Here's how the part is built. I have some questions about the finished solid (model axes, mm). A direction names the side the tool comes from. Coordinates: 2 decimals unless noted, no trailing zeros. Write each loop counter-clockwise with the first axis right and the second up, starting at its lowest first coordinate (ties: lowest second). Pieces come first, ordered by that corner, then holes.
Item 1: I'm going to push flat-ended pins straight in: P1, Ø5, axis at x = -108, z = -46.5, coming from the +Y side; P2, Ø12, axis at y = -65.5, z = -42, coming from the +X side; P3, Ø1.8, axis at x = -113, y = -22.5, coming from the +Z side; P4, Ø5, axis at x = -15.5, z = -22.5, coming from the +Y side. Where does each tip first touch, or does it pass through?
Item 2: I want a section at C-C (y = -14). Please give me the cut outline in (x, z), and give its area (3 significant figures).
Item 3: I want a section at A-A (z = -36). Count the separate pieces of the cut face and the enclosed holes in it, and give its area (3 significant figures).
Item 4: For faces 4 (the face through (-70, -11, -65)), 5 (the face through (-134, -3, -35)), 6 (the face through (-131, -12, -43)), 7 (the face through (-99, -1.8, -62)), 8 (the face through (-73.6, -61.9, -29.09)), which set-ups out of +Z, -Z, +X, -X, +Y, -Y let a thin tool reach every point of the face, with its end or its side?
Item 5: I want a section at B-B (x = -50). Please give me the cut outline in (y, z).
Item 6: I want a section at D-D (y = -44). Please give me the cut outline in (x, z), and give its area (3 significant figures).
Item 7: Please list where these lines run through material, in increasing order: line 1 (Y direction, x = -127, z = -37.5); line 2 (X direction, y = -7, z = -15); line 3 (Z direction, x = -83, y = -13).
Item 8: If we mould it in two halves opening along Y, with no side actions, what happens to faces 1 (the face through (-73, -18.5, -33)), 2 (the face through (0, -10, -35)), 3 (the face through (-68, 0, -37))? For each: pulls with the +Y half, pulls with the -Y half, needs draft (parallel to the pull), parting line crosses it, or undercut.
from build123d import *

# Parameters (mm, degrees)
MAIN_BODY_DEPTH     = 16
SKETCH8_W           = 134
SKETCH8_H           = 4
COVER_DEPTH         = 72
SKETCH20_W          = 116
SKETCH20_H          = 14
CRYSTAL_SLOT_DEPTH  = 65
SKETCH9_W           = 14
SKETCH9_H           = 14
SIPM_WINDOW_DEPTH   = 7
SKETCH10_R          = 23
SKETCH10_R_2        = 20
TUBE_ADAPTER_DEPTH  = 85
SKETCH21_W          = 54
SKETCH21_H          = 54
FILTER_SLOT_DEPTH   = 2.7
SKETCH24_W          = 49
SKETCH24_H          = 49
FILTER_WINDOW_DEPTH = 1.8
WIRE_SLOT_REACH     = 146
SKETCH25_W          = 25
SKETCH25_H          = 9


with BuildPart() as part:
    # Sketch5 → Main Body (new body)
    with BuildSketch(Plane(origin=(0, 0, 0), x_dir=(1, 0, 0), z_dir=(0, 1, 0))):
        Polygon((-134, 0), (-124, 0), (-1.95326153, 0), (0, 0), (0, 72), (-134, 72), align=None)
    extrude(amount=-MAIN_BODY_DEPTH)

    # Sketch8 → Cover (add)
    with BuildSketch(Plane.XY):
        with Locations((-67, -18)):
            Rectangle(SKETCH8_W, SKETCH8_H)
    extrude(amount=-COVER_DEPTH)

    # Sketch20 → Crystal Slot (cut)
    with BuildSketch(Plane.XY):
        with Locations((-69, -11.5)):
            Rectangle(SKETCH20_W, SKETCH20_H)
    extrude(amount=-CRYSTAL_SLOT_DEPTH, mode=Mode.SUBTRACT)

    # Sketch9 → SiPM Window (cut)
    with BuildSketch(Plane.ZY.offset(134)):
        with Locations((-36, -11.5)):
            Rectangle(SKETCH9_W, SKETCH9_H)
    extrude(amount=-SIPM_WINDOW_DEPTH, mode=Mode.SUBTRACT)

    # Sketch10 → Tube Adapter (add)
    with BuildSketch(Plane.XZ.offset(20)):
        with Locations((-95.536800003, -36)):
            Circle(SKETCH10_R)
        with Locations((-95.536800003, -36)):
            Circle(SKETCH10_R_2, mode=Mode.SUBTRACT)
    extrude(amount=TUBE_ADAPTER_DEPTH)

    # Sketch21 → Filter Slot (cut)
    with BuildSketch(Plane.XZ.offset(4.5)):
        with Locations((-40.5, -36)):
            Rectangle(SKETCH21_W, SKETCH21_H)
        with Locations((-97, -36)):
            Rectangle(SKETCH21_W, SKETCH21_H)
    extrude(amount=-FILTER_SLOT_DEPTH, mode=Mode.SUBTRACT)

    # Sketch24 → Filter Window (cut)
    with BuildSketch(Plane.XZ.offset(1.8)):
        with Locations((-40.5, -36)):
            Rectangle(SKETCH24_W, SKETCH24_H)
        with Locations((-97, -36)):
            Rectangle(SKETCH24_W, SKETCH24_H)
    extrude(amount=-FILTER_WINDOW_DEPTH, mode=Mode.SUBTRACT)

    # Sketch25 → Wire Slot (cut, up to next)
    with BuildSketch(Plane.ZY.offset(144), mode=Mode.PRIVATE) as wire_slot_sk1:
        with Locations((-36, -24.5)):
            Rectangle(SKETCH25_W, SKETCH25_H)
    wire_slot_tool1 = extrude(wire_slot_sk1.sketch, amount=-WIRE_SLOT_REACH, mode=Mode.PRIVATE) & part.part
    add(wire_slot_tool1.solids().sort_by_distance((-144, -24.5, -36))[0], mode=Mode.SUBTRACT)


solid = part.part
Answer:
1. P1: stops at y = -18.5
1. P2: stops at x = -72.54
1. P3: stops at z = -20.04
1. P4: stops at y = 0
2. outline: (-134, -72) - (0, -72) - (0, 0) - (-11, 0) - (-11, -65) - (-127, -65) - (-127, -43) - (-134, -43) - close; (-134, -29) - (-127, -29) - (-127, 0) - (-134, 0) - close
2. area: 2,010 mm2
3. separate pieces: 4
3. enclosed holes: 0
3. area: 973 mm2
4. face 4: +Z
4. face 5: +Z, -Z, -X, +Y, -Y
4. face 6: -X
4. face 7: none
4. face 8: -Y
5. outline: (-20, -72) - (0, -72) - (0, -60.5) - (-1.8, -60.5) - (-1.8, -63) - (-4.5, -63) - (-4.5, -65) - (-18.5, -65) - (-18.5, 0) - (-20, 0) - close; (-4.5, -9) - (-1.8, -9) - (-1.8, -11.5) - (0, -11.5) - (0, 0) - (-4.5, 0) - close
6. outline: circle Ø46 at (-95.54, -36); hole circle Ø40 at (-95.54, -36)
6. area: 405 mm2
7. line 1: y = -20 to -18.5, -4.5 to 0
7. line 2: x = -134 to -127, -11 to 0
7. line 3: z = -72 to -65
8. face 1: undercut
8. face 2: needs draft
8. face 3: pulls with the +Y half
